```python
from build123d import *

# Parameters (mm, degrees)
SALIENTE_EXTRUIR1_DEPTH      = 40
SALIENTE_EXTRUIR1_DEPTH_BACK = 40
CROQUIS1_R                   = 44.5
CORTAR_EXTRUIR1_DEPTH        = 35
CORTAR_EXTRUIR1_DEPTH_BACK   = 35
CROQUIS2_OUTSIDE_W           = 120.828
CROQUIS2_OUTSIDE_H           = 120.828
CORTAR_EXTRUIR2_REACH        = 99.906
CROQUIS3_R                   = 5.5
SALIENTE_EXTRUIR2_START      = 15
CROQUIS4_R                   = 7.5
SALIENTE_EXTRUIR2_DEPTH      = 15


with BuildPart() as part:
    # Croquis1 → Saliente-Extruir1 (new, two sides: drawn at the far end of the back side and taken through both)
    with BuildSketch(Plane(origin=(0, 0, 0), x_dir=(1, 0, 0), z_dir=(0, 1, 0)).offset(-SALIENTE_EXTRUIR1_DEPTH_BACK)):
        with Locations(Location((0, 0, 0), (0, 0, 270))):
            Circle(CROQUIS1_R)
    extrude(amount=SALIENTE_EXTRUIR1_DEPTH + SALIENTE_EXTRUIR1_DEPTH_BACK)

    # Croquis2 outside → Cortar-Extruir1 (cut, two sides: drawn at the far end of the back side and taken through both)
    with BuildSketch(Plane(origin=(0, 0, 0), x_dir=(1, 0, 0), z_dir=(0, 1, 0)).offset(-CORTAR_EXTRUIR1_DEPTH_BACK)):
        Rectangle(CROQUIS2_OUTSIDE_W, CROQUIS2_OUTSIDE_H)
        with BuildLine():
            Line((35.739256, 9.576305), (42.983699, 11.517448))
            ThreePointArc((42.983699, 11.517448), (44.5, 0), (42.983699, -11.517448))
            Line((42.983699, -11.517448), (35.739256, -9.576305))
            ThreePointArc((35.739256, -9.576305), (37, 0), (35.739256, 9.576305))
        make_face(mode=Mode.SUBTRACT)
        with BuildLine():
            Line((-35.739256, -9.576305), (-42.983699, -11.517448))
            ThreePointArc((-42.983699, -11.517448), (-44.5, 0), (-42.983699, 11.517448))
            Line((-42.983699, 11.517448), (-35.739256, 9.576305))
            ThreePointArc((-35.739256, 9.576305), (-37, 0), (-35.739256, -9.576305))
        make_face(mode=Mode.SUBTRACT)
    extrude(amount=CORTAR_EXTRUIR1_DEPTH + CORTAR_EXTRUIR1_DEPTH_BACK, mode=Mode.SUBTRACT)

    # Croquis3 → Cortar-Extruir2 (cut, up to next)
    with BuildSketch(Plane(origin=(0, -35, 0), x_dir=(1, 0, 0), z_dir=(0, 1, 0)), mode=Mode.PRIVATE) as cortar_extruir2_sk1:
        with Locations(Location((0, 0, 0), (0, 0, 270))):
            Circle(CROQUIS3_R)
    cortar_extruir2_tool1 = extrude(cortar_extruir2_sk1.sketch, amount=-CORTAR_EXTRUIR2_REACH, mode=Mode.PRIVATE) & part.part
    # Croquis3 → Cortar-Extruir2 (cut, up to next)
    with BuildSketch(Plane(origin=(0, -35, 0), x_dir=(1, 0, 0), z_dir=(0, 1, 0)), mode=Mode.PRIVATE) as cortar_extruir2_sk2:
        with BuildLine():
            Line((42.983699, 11.517448), (7.244444, 1.941143))
            ThreePointArc((7.244444, 1.941143), (0, 7.5), (-7.244444, 1.941143))
            Line((-7.244444, 1.941143), (-42.983699, 11.517448))
            ThreePointArc((-42.983699, 11.517448), (0, 44.5), (42.983699, 11.517448))
        make_face()
    cortar_extruir2_tool2 = extrude(cortar_extruir2_sk2.sketch, amount=-CORTAR_EXTRUIR2_REACH, mode=Mode.PRIVATE) & part.part
    # Croquis3 → Cortar-Extruir2 (cut, up to next)
    with BuildSketch(Plane(origin=(0, -35, 0), x_dir=(1, 0, 0), z_dir=(0, 1, 0)), mode=Mode.PRIVATE) as cortar_extruir2_sk3:
        with BuildLine():
            Line((42.983699, -11.517448), (7.244444, -1.941143))
            ThreePointArc((7.244444, -1.941143), (0, -7.5), (-7.244444, -1.941143))
            Line((-7.244444, -1.941143), (-42.983699, -11.517448))
            ThreePointArc((-42.983699, -11.517448), (0, -44.5), (42.983699, -11.517448))
        make_face()
    cortar_extruir2_tool3 = extrude(cortar_extruir2_sk3.sketch, amount=-CORTAR_EXTRUIR2_REACH, mode=Mode.PRIVATE) & part.part
    add(cortar_extruir2_tool1.solids().sort_by_distance((0, -35, 0))[0], mode=Mode.SUBTRACT)
    add(cortar_extruir2_tool2.solids().sort_by_distance((0, -35, -22.423567))[0], mode=Mode.SUBTRACT)
    add(cortar_extruir2_tool3.solids().sort_by_distance((0, -35, 22.423567))[0], mode=Mode.SUBTRACT)

    # Croquis4 → Saliente-Extruir2 (add)
    with BuildSketch(Plane(origin=(0, 40, 0), x_dir=(1, 0, 0), z_dir=(0, 1, 0)).offset(SALIENTE_EXTRUIR2_START)):
        with Locations(Location((0, 0, 0), (0, 0, 270))):
            Circle(CROQUIS4_R)
    extrude(amount=-SALIENTE_EXTRUIR2_DEPTH)


solid = part.part
```
Source: CAD feature listing. Evaluate the final solid. Frame: model axes, mm. A direction names the side the tool comes from. Give positions to 0.01 mm unless a question says otherwise; leave off trailing zeros. Loops run counter-clockwise (first coordinate to the right, second up) from the corner with the lowest first, then second, coordinate; pieces in that order, holes last. Notation, with made-up numbers: (30, 5) -> (61, 5) arc R35 cw to (61, 43) -> close; hole circle Ø9 at (67.25, 80.25). An arc over 180 degrees is marked (long way). Use a Markdown table: item, result. Add a question column.
(1) First-contact query: pin 1 Ø6 at (x, z) = (9, 32) entering from +Y; pin 2 Ø9 at (x, z) = (0, 0) entering from -Y; pin 3 Ø6 at (x, y) = (18.5, 42.5) entering from +Z. Flat tips, straight axial feed; report the tip coordinate or a pass-through.
(2) Pull-direction query (Z, two-part tool) for faces 5 (the face through (-37, 0, 0)), 6 (the face through (0.1, -37.5, 7.5)), 7 (the face through (0.33, 47.605, -7.493)); classes: +Z half, -Z half, draft (parallel to the pull), parting line (faces both ways), or undercut.
(3) Section query B-B (x = 13.5). Output: boundary loops of the cut face in (y, z).
(4) Access query for faces 1 (the face through (37, 0, 0)), 2 (the face through (11, -40, 0)), 3 (the face through (-5.37, -37.47, -1.19)), 4 (the face through (0.1, -37.5, -7.5)). Directions: +Z, -Z, +X, -X, +Y, -Y. A direction counts if a zero-diameter tool reaches every point of the face in a straight line with its end or side. Return the directions, or none.
(5) Section query C-C (x = 0). Output: boundary loops of the cut face in (y, z), then the cut area to 3 significant figures.
(6) Section query D-D (z = 0). Output: boundary loops of the cut face in (x, y).
(7) Section query A-A (y = -23). Output: boundary loops of the cut face in (x, z), then the cut area to 3 significant figures.
(8) Ray query, line 1 (X direction, y = -38.75, z = 0); line 2 (Y direction, x = 22, z = -26); line 3 (Y direction, x = 31.5, z = 0). Return the intervals inside material, ascending.
Checked values:
| question | item | result |
|---|---|---|
| 1 | pin 1 | y = 40 |
| 1 | pin 2 | y = 35 |
| 1 | pin 3 | z = 41.19 |
| 2 | face 5 | undercut |
| 2 | face 6 | +Z half |
| 2 | face 7 | parting line |
| 3 | outline | (-40, -3.62) -> (-35, -3.62) -> (-35, 3.62) -> (-40, 3.62) -> close; (35, -42.4) -> (40, -42.4) -> (40, 42.4) -> (35, 42.4) -> close |
| 4 | face 1 | none |
| 4 | face 2 | +Z, -Z, +X, -X, -Y |
| 4 | face 3 | -Y |
| 4 | face 4 | -Z, -Y |
| 5 | outline | (-40, -7.5) -> (-35, -7.5) -> (-35, -5.5) -> (-40, -5.5) -> close; (-40, 5.5) -> (-35, 5.5) -> (-35, 7.5) -> (-40, 7.5) -> close; (35, -44.5) -> (40, -44.5) -> (40, -7.5) -> (55, -7.5) -> (55, 7.5) -> (40, 7.5) -> (40, 44.5) -> (35, 44.5) -> close |
| 5 | area | 690 mm^2 |
| 6 | outline | (-44.5, -40) -> (-5.5, -40) -> (-5.5, -35) -> (-37, -35) -> (-37, 35) -> (37, 35) -> (37, -35) -> (5.5, -35) -> (5.5, -40) -> (44.5, -40) -> (44.5, 40) -> (7.5, 40) -> (7.5, 55) -> (-7.5, 55) -> (-7.5, 40) -> (-44.5, 40) -> close |
| 7 | outline | (-42.98, -11.52) -> (-35.74, -9.58) arc R37 cw to (-35.74, 9.58) -> (-42.98, 11.52) arc R44.5 ccw to start; (35.74, -9.58) -> (42.98, -11.52) arc R44.5 ccw to (42.98, 11.52) -> (35.74, 9.58) arc R37 cw to start |
| 7 | area | 320 mm^2 |
| 8 | line 1 | -44.5 to -5.5, 5.5 to 44.5 |
| 8 | line 2 | 35 to 40 |
| 8 | line 3 | -40 to -35, 35 to 40 |
